Study the drawing (mm; zero at the part's minimum x, y, z) and answer. Coordinates: 2 decimals unless noted, no trailing zeros. Order: outer loops, then holes, each group sorted by start corner. A loop starts at its lowest first (then second) coordinate and runs counter-clockwise, first axis right, second up. Notation, with made-up numbers: (5, 8.25) - (60, 8.25) arc R24 cw to (60, 41.25) - close; hole circle Ø9 at (22.25, 86.5). An arc over 180 degrees is marked (long way). Write item = value, one per line.
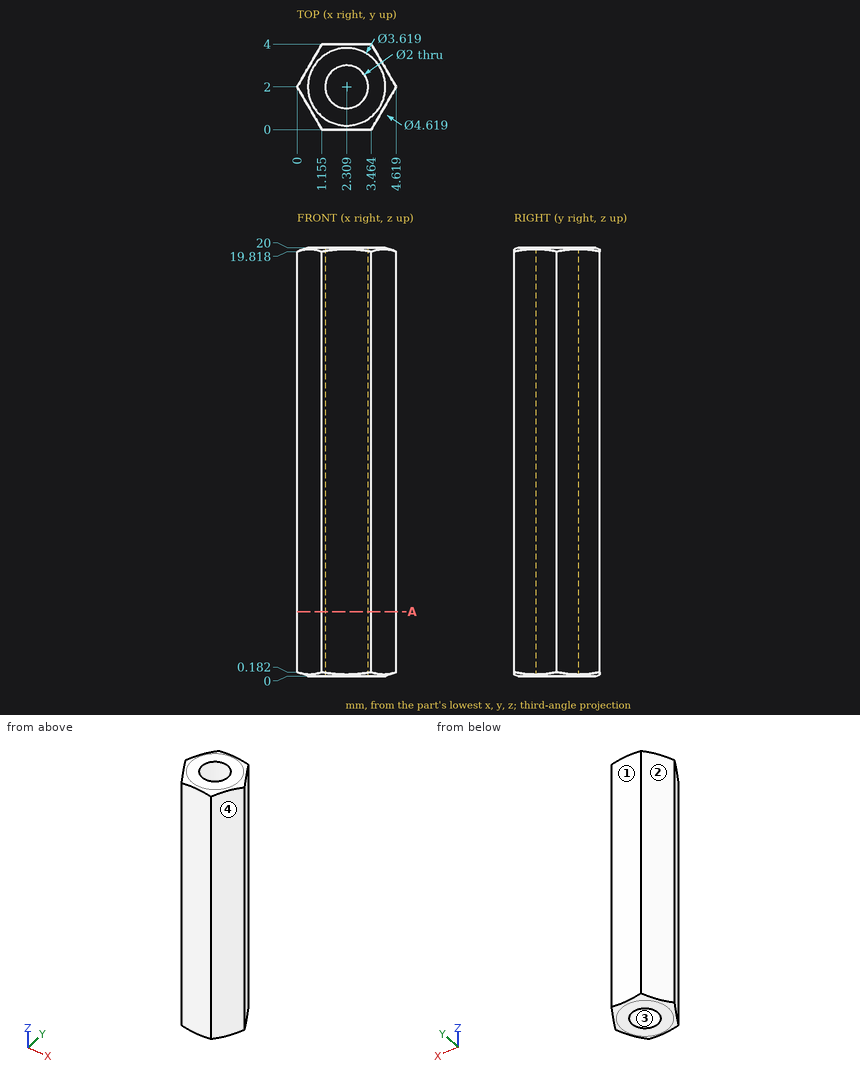
1) A flat-ended cylindrical pin translates along its axis: pin 1 Ø1 at (x, z) = (3.5, 12) entering from -Y. Find the tip coordinate at first contact, or state that the pin passes through.
Returned:
pin_1 = 0
2) Straight lines are drawn through the part: line 1 along Y through (x, z) = (2.9, 8.5) (1 decimal); line 2 along X through (y, z) = (1.65, 10) (1 decimal); line 3 along Z through (x, y) = (1.65, 3.7) (1 decimal). For each, find the intervals that lie inside material, in ascending order. Write a range as from..to.
Returned:
line_1 = 0..1.2, 2.8..4
line_2 = 0.2..1.4, 3.2..4.4
line_3 = 0..20
3) Determine the mould class of the marked faces 1, 2, 3 and 4 for opening direction X: pulls with the +X half, pulls with the -X half, needs draft (parallel to the pull), parting line crosses it, or undercut.
Returned:
face_1 = needs draft
face_2 = pulls with the -X half
face_3 = undercut
face_4 = pulls with the +X half
4) The part is cut by section A-A (z = 3). Determine the outline of the cut face in (x, y) (1 decimal), and give its area (3 significant figures).
Returned:
outline = (0, 2) - (1.2, 0) - (3.5, 0) - (4.6, 2) - (3.5, 4) - (1.2, 4) - close; hole circle Ø2 at (2.3, 2)
area = 10.7 mm^2
